The drawing under review shows one solid part. Ordinate dimensions are in mm from its lowest x, y, z. Coordinates: 2 decimals unless noted, no trailing zeros. Loops run counter-clockwise (first coordinate to the right, second up) from the corner with the lowest first, then second, coordinate; pieces in that order, holes last. Notation, with made-up numbers: (-28, 28) -> (8, 28) arc R7 cw to (8, 41) -> close; hole circle Ø5 at (18, 54.25). An arc over 180 degrees is marked (long way). Use a Markdown table: item, result.
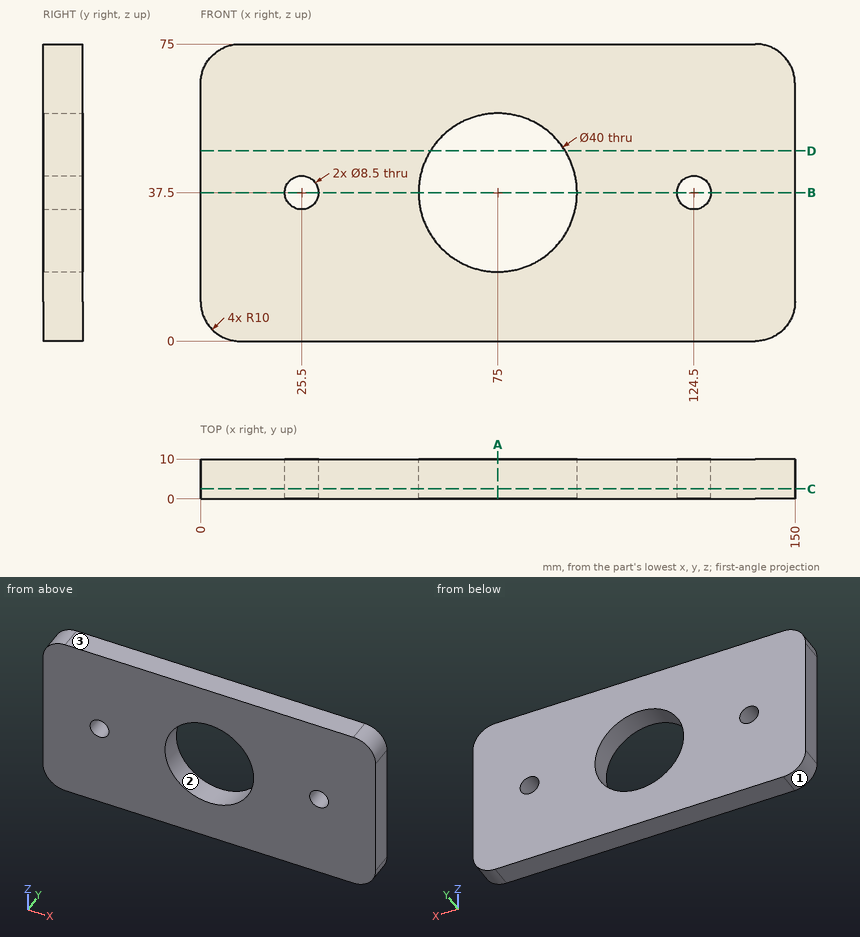
(1) Mouldability with a two-part tool opening along X and no side actions: class the marked faces 1, 2 and 3 as pulls with the +X half, pulls with the -X half, needs draft (parallel to the pull), parting line crosses it, or undercut.
Found:
| item | result |
|---|---|
| face 1 | pulls with the -X half |
| face 2 | undercut |
| face 3 | needs draft |
(2) Take a section at A-A on x = 75. Write out the cut boundary in (y, z).
Found:
| item | result |
|---|---|
| outline | (0, 0) -> (10, 0) -> (10, 17.5) -> (0, 17.5) -> close; (0, 57.5) -> (10, 57.5) -> (10, 75) -> (0, 75) -> close |
(3) Take a section at C-C on y = 2.5. Write out the cut boundary in (x, z).
Found:
| item | result |
|---|---|
| outline | (0, 10) arc R10 ccw to (10, 0) -> (140, 0) arc R10 ccw to (150, 10) -> (150, 65) arc R10 ccw to (140, 75) -> (10, 75) arc R10 ccw to (0, 65) -> close; hole circle Ø8.5 at (25.5, 37.5); hole circle Ø40 at (75, 37.5); hole circle Ø8.5 at (124.5, 37.5) |
(4) Take a section at D-D on z = 48. Write out the cut boundary in (x, y), plus the area to 3 significant figures.
Found:
| item | result |
|---|---|
| outline | (0, 0) -> (57.98, 0) -> (57.98, 10) -> (0, 10) -> close; (92.02, 0) -> (150, 0) -> (150, 10) -> (92.02, 10) -> close |
| area | 1,160 mm^2 |
(5) For line 1 along Z through (x, y) = (25.5, 3.25); line 2 along Z through (x, y) = (75, 3); line 3 along X through (y, z) = (1.25, 29), list the stretches that pass through material, from the lowest coordinate up.
Found:
| item | result |
|---|---|
| line 1 | z = 0 to 33.25, 41.75 to 75 |
| line 2 | z = 0 to 17.5, 57.5 to 75 |
| line 3 | x = 0 to 56.9, 93.1 to 150 |
(6) Take a section at B-B on z = 37.5. Write out the cut boundary in (x, y).
Found:
| item | result |
|---|---|
| outline | (0, 0) -> (21.25, 0) -> (21.25, 10) -> (0, 10) -> close; (29.75, 0) -> (55, 0) -> (55, 10) -> (29.75, 10) -> close; (95, 0) -> (120.25, 0) -> (120.25, 10) -> (95, 10) -> close; (128.75, 0) -> (150, 0) -> (150, 10) -> (128.75, 10) -> close |
(7) For pin 1 Ø24 at (x, z) = (75, 37.5) entering from +Y, flat-tipped, find the tip position at first contact; note if it passes through.
Found:
| item | result |
|---|---|
| pin 1 | passes through |
